Can you work these out from the model? Positions are in its coordinate system, mm. Face numbers are marked on the shaded views. Give positions to 0.01 mm unless a question says otherwise; leave off trailing zeros. Order: outer loops, then holes, each group sorted by start corner. A loop starts at its lowest first (then second) coordinate and runs counter-clockwise, first axis right, second up.
Item 1: I want a section at B-B, the plane x = -127. Write out the boundary of the cut face in (y, z), then the cut area to 3 significant figures.
Item 2: If we mould it in two halves opening along X, with no side actions, what happens to the marked faces 1 and 2? For each: +X half, -X half, draft (parallel to the pull), parting line (faces both ways), or undercut.
Item 3: I want a section at D-D, the plane y = 72. Write out the boundary of the cut face in (x, z), then the cut area to 3 significant figures.
Item 4: I want a section at C-C, the plane z = 5.75. Write out the boundary of the cut face in (x, y).
Item 5: If I drill on line 1 along X through (y, z) = (111, 0.75); line 2 along Y through (x, z) = (-133, 7); line 3 along Y through (x, z) = (-126, 6.25), over which ranges is the centre line in solid material (lowest first)?
Item 6: I want a section at A-A, the plane y = 103.5. Write out the boundary of the cut face in (x, z).
```python
from build123d import *

# Parameters (mm, degrees)
SKETCH1_W           = 40
SKETCH1_H           = 160
BOSS_EXTRUDE1_DEPTH = 10
SKETCH2_R           = 10
CUT_EXTRUDE1_DEPTH  = 11
LPATTERN1_COUNT     = 4
LPATTERN1_PITCH     = 36


with BuildPart() as part:
    # Sketch1 → Boss-Extrude1 (new body)
    with BuildSketch(Plane.XY):
        with Locations((-128.294392523, 130.11682243)):
            Rectangle(SKETCH1_W, SKETCH1_H)
    extrude(amount=BOSS_EXTRUDE1_DEPTH)

    # Sketch2 → Cut-Extrude1 (cut, through all)
    with BuildSketch(Plane.XY.offset(10)):
        with Locations((-128.294392523, 75.11682243)):
            Circle(SKETCH2_R)
    cut_extrude1 = extrude(amount=-CUT_EXTRUDE1_DEPTH, mode=Mode.SUBTRACT)

    # LPattern1: Cut-Extrude1 ×4
    with Locations(*[(0, i * LPATTERN1_PITCH, 0) for i in range(1, LPATTERN1_COUNT)]):
        add(cut_extrude1, mode=Mode.SUBTRACT)


solid = part.part
```
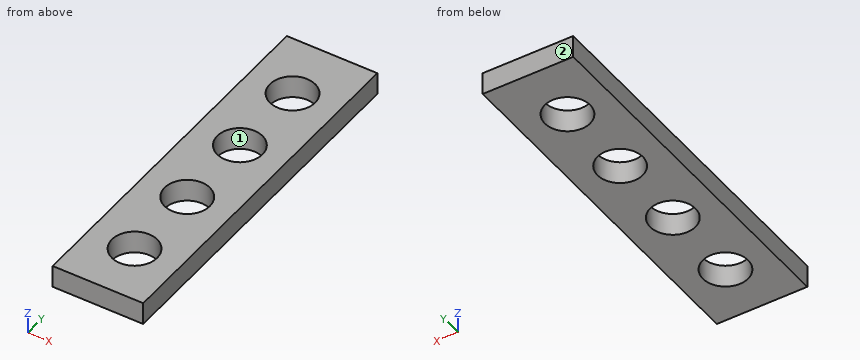
Results list:
1. outline: (50.12, 0) - (65.2, 0) - (65.2, 10) - (50.12, 10) - close; (85.03, 0) - (101.2, 0) - (101.2, 10) - (85.03, 10) - close; (121.03, 0) - (137.2, 0) - (137.2, 10) - (121.03, 10) - close; (157.03, 0) - (173.2, 0) - (173.2, 10) - (157.03, 10) - close; (193.03, 0) - (210.12, 0) - (210.12, 10) - (193.03, 10) - close
1. area: 807 mm2
2. face 1: undercut
2. face 2: draft
3. outline: (-148.29, 0) - (-137.8, 0) - (-137.8, 10) - (-148.29, 10) - close; (-118.79, 0) - (-108.29, 0) - (-108.29, 10) - (-118.79, 10) - close
3. area: 210 mm2
4. outline: (-148.29, 50.12) - (-108.29, 50.12) - (-108.29, 210.12) - (-148.29, 210.12) - close; hole circle Ø20 at (-128.29, 75.12); hole circle Ø20 at (-128.29, 111.12); hole circle Ø20 at (-128.29, 147.12); hole circle Ø20 at (-128.29, 183.12)
5. line 1: x = -148.29 to -138.29, -118.3 to -108.29
5. line 2: y = 50.12 to 66.29, 83.94 to 102.29, 119.94 to 138.29, 155.94 to 174.29, 191.94 to 210.12
5. line 3: y = 50.12 to 65.38, 84.85 to 101.38, 120.85 to 137.38, 156.85 to 173.38, 192.85 to 210.12
6. outline: (-148.29, 0) - (-134.77, 0) - (-134.77, 10) - (-148.29, 10) - close; (-121.81, 0) - (-108.29, 0) - (-108.29, 10) - (-121.81, 10) - close
